Design review of the part shown in the three views and the two pictorial views. Dimensions are in mm from the part's minimum x, y and z. A direction names the side the tool comes from. Round coordinates to 2 decimals unless told otherwise and drop trailing zeros. One line per question, with ' | ' between items. Start each with the question number.
1. Draft analysis for pull direction Y (two halves, no side actions). For the marked faces 1, 2 and 3, state which applies: pulls with the +Y half, pulls with the -Y half, needs draft (parallel to the pull), parting line crosses it, or undercut.
2. Wall thickness on line 1 along Y through (x, z) = (11, 6) (1 decimal); line 2 along X through (y, z) = (8.75, 4.5) (1 decimal): over which ranges is each line inside the solid? List them lowest first.
3. For pin 1 Ø1.5 at (y, z) = (6, 3.5) entering from +X (1 decimal); pin 2 Ø1.5 at (y, z) = (10, 3) entering from -X; pin 3 Ø4 at (x, z) = (14, 6) entering from -Y, all flat-tipped, find the tip position at first contact; note any pin that passes through.
4. For the marked faces 4 and 5, list the 3-axis set-ups (+Z, -Z, +X, -X, +Y, -Y) from which the entire face can be reached by the end or side of a thin tool; tool diameter is ignored.
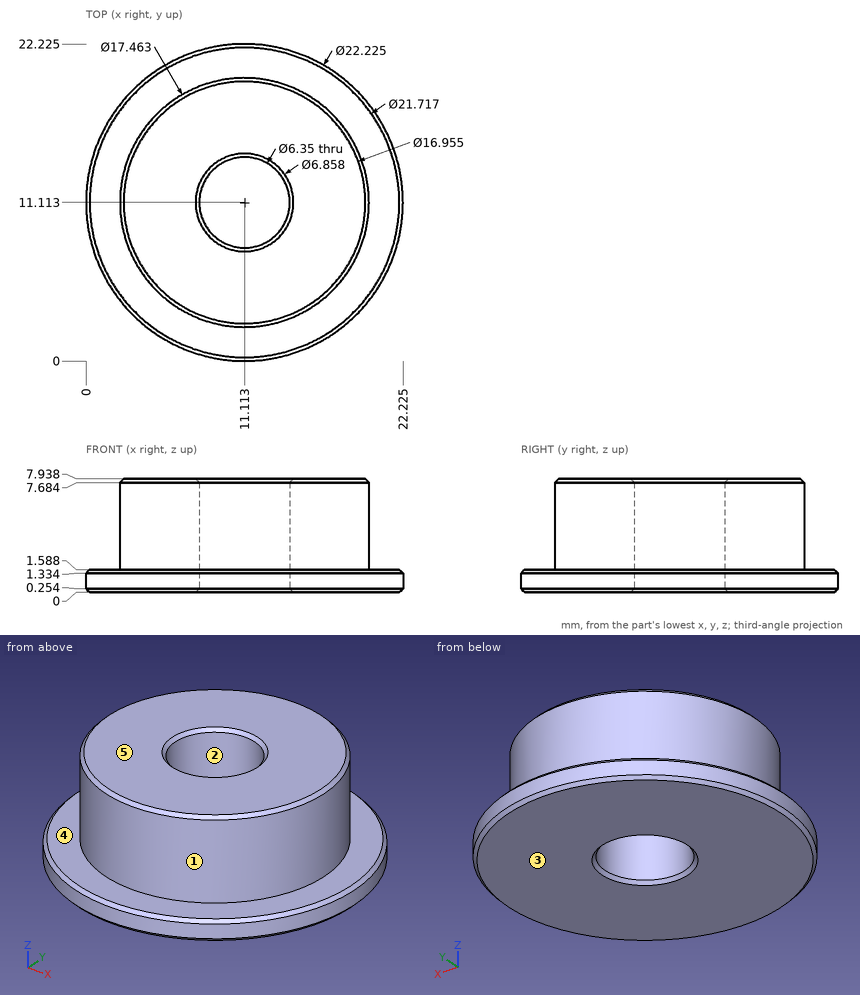
Answer block:
1) face 1: parting line crosses it | face 2: undercut | face 3: needs draft
2) line 1: y = 2.4 to 7.9, 14.3 to 19.8 | line 2: x = 2.7 to 9, 13.2 to 19.5
3) pin 1: stops at x = 18.7 | pin 2: stops at x = 2.39 | pin 3: stops at y = 2.43
4) face 4: +Z | face 5: +Z, +X, -X, +Y, -Y
